from build123d import *

# Parameters (mm, degrees)
SKETCH1_W           = 60
SKETCH1_H           = 95
BOSS_EXTRUDE1_DEPTH = 1
SKETCH2_W           = 5
SKETCH2_H           = 26
BOSS_EXTRUDE2_DEPTH = 8.5
CUT_EXTRUDE1_REACH  = 58.978
SKETCH3_R           = 1.5


with BuildPart() as part:
    # Sketch1 → Boss-Extrude1 (new body)
    with BuildSketch(Plane(origin=(0, 0, 0), x_dir=(1, 0, 0), z_dir=(0, 1, 0))):
        Rectangle(SKETCH1_W, SKETCH1_H)
    extrude(amount=BOSS_EXTRUDE1_DEPTH)

    # Sketch2 → Boss-Extrude2 (add)
    with BuildSketch(Plane.XZ):
        with Locations((21.75, 14.5)):
            Rectangle(SKETCH2_W, SKETCH2_H)
        with Locations((-21.75, 14.5)):
            Rectangle(SKETCH2_W, SKETCH2_H)
    extrude(amount=BOSS_EXTRUDE2_DEPTH)

    # Sketch3 → Cut-Extrude1 (cut, up to next)
    with BuildSketch(Plane(origin=(0, 1, 0), x_dir=(1, 0, 0), z_dir=(0, 1, 0)), mode=Mode.PRIVATE) as cut_extrude1_sk1:
        with Locations(Location((-27, -45, 0), (0, 0, 270))):
            Circle(SKETCH3_R)
    cut_extrude1_tool1 = extrude(cut_extrude1_sk1.sketch, amount=-CUT_EXTRUDE1_REACH, mode=Mode.PRIVATE) & part.part
    # Sketch3 → Cut-Extrude1 (cut, up to next)
    with BuildSketch(Plane(origin=(0, 1, 0), x_dir=(1, 0, 0), z_dir=(0, 1, 0)), mode=Mode.PRIVATE) as cut_extrude1_sk2:
        with Locations(Location((27, -45, 0), (0, 0, 270))):
            Circle(SKETCH3_R)
    cut_extrude1_tool2 = extrude(cut_extrude1_sk2.sketch, amount=-CUT_EXTRUDE1_REACH, mode=Mode.PRIVATE) & part.part
    # Sketch3 → Cut-Extrude1 (cut, up to next)
    with BuildSketch(Plane(origin=(0, 1, 0), x_dir=(1, 0, 0), z_dir=(0, 1, 0)), mode=Mode.PRIVATE) as cut_extrude1_sk3:
        with Locations(Location((27, 45, 0), (0, 0, 270))):
            Circle(SKETCH3_R)
    cut_extrude1_tool3 = extrude(cut_extrude1_sk3.sketch, amount=-CUT_EXTRUDE1_REACH, mode=Mode.PRIVATE) & part.part
    # Sketch3 → Cut-Extrude1 (cut, up to next)
    with BuildSketch(Plane(origin=(0, 1, 0), x_dir=(1, 0, 0), z_dir=(0, 1, 0)), mode=Mode.PRIVATE) as cut_extrude1_sk4:
        with Locations(Location((-27, 45, 0), (0, 0, 270))):
            Circle(SKETCH3_R)
    cut_extrude1_tool4 = extrude(cut_extrude1_sk4.sketch, amount=-CUT_EXTRUDE1_REACH, mode=Mode.PRIVATE) & part.part
    add(cut_extrude1_tool1.solids().sort_by_distance((-27, 1, 45))[0], mode=Mode.SUBTRACT)
    add(cut_extrude1_tool2.solids().sort_by_distance((27, 1, 45))[0], mode=Mode.SUBTRACT)
    add(cut_extrude1_tool3.solids().sort_by_distance((27, 1, -45))[0], mode=Mode.SUBTRACT)
    add(cut_extrude1_tool4.solids().sort_by_distance((-27, 1, -45))[0], mode=Mode.SUBTRACT)


solid = part.part
Design review of the part built by this model. Coordinates are the model's own, in mm. A direction names the side the tool comes from. Round coordinates to 2 decimals unless told otherwise and drop trailing zeros. Write each loop counter-clockwise with the first axis right and the second up, starting at its lowest first coordinate (ties: lowest second). Pieces come first, ordered by that corner, then holes. Notation, with made-up numbers: (-20.75, 38.5) -> (4.25, 38.5) arc R25 ccw to (4.25, 58.5) -> close; hole circle Ø2 at (10.25, 24.5). An arc over 180 degrees is marked (long way). One line per question, with ' | ' between items.
(1) Draft analysis for pull direction Z (two halves, no side actions). For faces 4 (the cylindrical face through (28.01, 0.51, -46.11)), 5 (the flat face through (19.25, -4, 14)), 6 (the flat face through (22, -4, 27.5)), state which applies: released by +Z, released by -Z, zero draft, split by the parting line, or undercut.
Result sheet:
face 4: undercut | face 5: zero draft | face 6: released by +Z
(2) Take a section at A-A, the plane z = -45. State the section outline as (x, y) points.
Result sheet:
outline: (-30, 0) -> (-28.5, 0) -> (-28.5, 1) -> (-30, 1) -> close; (-25.5, 0) -> (25.5, 0) -> (25.5, 1) -> (-25.5, 1) -> close; (28.5, 0) -> (30, 0) -> (30, 1) -> (28.5, 1) -> close
(3) Take a section at B-B, the plane x = 27. State the section outline as (y, z) points, and give its area (3 significant figures).
Result sheet:
outline: (0, -47.5) -> (1, -47.5) -> (1, -46.5) -> (0, -46.5) -> close; (0, -43.5) -> (1, -43.5) -> (1, 43.5) -> (0, 43.5) -> close; (0, 46.5) -> (1, 46.5) -> (1, 47.5) -> (0, 47.5) -> close | area: 89.0 mm2
(4) Machinability: for faces 1 (the flat face through (-19.25, -4, 14)), 2 (the flat face through (-24.25, -4, 14)), 3 (the flat face through (-22, -4, 1.5)), which of the approach directions +Z, -Z, +X, -X, +Y, -Y give a long, thin tool a straight path to every point of the face, cutting with its end or side? Answer none if there is none.
Result sheet:
face 1: +Z, -Z, -Y | face 2: +Z, -Z, -X, -Y | face 3: -Z, +X, -X, -Y
(5) Wall thickness on line 1 (X direction, y = 0.7, z = -45); line 2 (X direction, y = -8, z = 12); line 3 (Y direction, x = 20, z = -4.5): over which ranges is each line inside the solid? List them lowest first. Write a range as [from, to].
Result sheet:
line 1: [-30, -28.5], [-25.5, 25.5], [28.5, 30] | line 2: [-24.25, -19.25], [19.25, 24.25] | line 3: [0, 1]
(6) Take a section at D-D, the plane x = -22. State the section outline as (y, z) points.
Result sheet:
outline: (-8.5, 1.5) -> (0, 1.5) -> (0, -47.5) -> (1, -47.5) -> (1, 47.5) -> (0, 47.5) -> (0, 27.5) -> (-8.5, 27.5) -> close
(7) Take a section at C-C, the plane y = -3.5. State the section outline as (x, z) points.
Result sheet:
outline: (-24.25, 1.5) -> (-19.25, 1.5) -> (-19.25, 27.5) -> (-24.25, 27.5) -> close; (19.25, 1.5) -> (24.25, 1.5) -> (24.25, 27.5) -> (19.25, 27.5) -> close
(8) Insertion check: P1, Ø2.5, axis at x = -21.5, y = -4.5, coming from the +Z side; P2, Ø5, axis at x = -27, z = -45, coming from the -Y side; P3, Ø2.5, axis at x = 27, z = 45, coming from the +Y side; P4, Ø4, axis at y = -4.5, z = 19.5, coming from the +X side. Each pin has a flat end and moves straight along its axis. Give the tip position at first contact, or say it passes through.
Result sheet:
P1: z = 27.5 | P2: y = 0 | P3: through | P4: x = 24.25
